The listing builds one solid part. Answer for the finished solid, in the listing's coordinates (mm). Coordinates: 2 decimals unless noted, no trailing zeros. Loops run counter-clockwise (first coordinate to the right, second up) from the corner with the lowest first, then second, coordinate; pieces in that order, holes last. Notation, with made-up numbers: (33, 3.5) - (61, 3.5) arc R12 cw to (61, 24.5) - close; hole circle Ø1 at (-39, 12.25). An arc over 180 degrees is marked (long way). One line per question, with ' | ' between items.
from build123d import *

# Parameters (mm, degrees)
F0_W     = 6.985
F0_H     = 1.5875
F1_DEPTH = 0.94615
F2_W     = 1.5875
F2_H     = 1.5875
F3_DEPTH = 4.445
F4_R     = 0.762


with BuildPart() as f1:
    # F0 (on Top) → F1 (new body)
    with BuildSketch(Plane.XY):
        with Locations((3.4925, 0.79375)):
            Rectangle(F0_W, F0_H)
    extrude(amount=F1_DEPTH)

    # F2 (on face) → F3 (join)
    with BuildSketch(Plane.XY.offset(0.94615)):
        with Locations((0.79375, 0.79375)):
            Rectangle(F2_W, F2_H)
        with Locations((6.19125, 0.79375)):
            Rectangle(F2_W, F2_H)
    extrude(amount=F3_DEPTH)

    # F4
    f4_edges = [f1.edges().sort_by_distance(p)[0] for p in [
        (0, 0, 2.695575),
        (1.5875, 0, 3.16865),
        (3.4925, 0, 0.94615),
        (5.3975, 0, 3.16865),
        (6.985, 0, 2.695575),
        (0, 1.5875, 2.695575),
        (1.5875, 1.5875, 3.16865),
        (3.4925, 1.5875, 0.94615),
        (5.3975, 1.5875, 3.16865),
        (6.985, 1.5875, 2.695575),
    ]]
    fillet(f4_edges, radius=F4_R)


solid = f1.part
Item 1: Find section C-C, the plane x = 4.5. Write down the section's boundary in (y, z), plus the area to 3 significant figures.
Taken from the geometry:
outline: (0, 0) - (1.59, 0) - (1.59, 0.18) arc R0.76 ccw to (0.83, 0.95) - (0.76, 0.95) arc R0.76 ccw to (0, 0.18) - close | area: 1.25 mm2
Item 2: Find section B-B, the plane y = 0.55. Write down the section's boundary in (x, z).
Taken from the geometry:
outline: (0.03, 0) - (6.95, 0) - (6.95, 5.39) - (5.43, 5.39) - (5.43, 0.92) - (1.56, 0.92) - (1.56, 5.39) - (0.03, 5.39) - close
Item 3: Find the intervals of material crossed by line 1 (X direction, y = 0.75, z = 4.8); line 2 (X direction, y = 1.4, z = 3.2); line 3 (Z direction, x = 3.5, y = 0.7), in increasing order. Write a range as [from, to].
Taken from the geometry:
line 1: x = [0, 1.59], [5.4, 6.98] | line 2: x = [0.26, 1.33], [5.66, 6.72] | line 3: z = [0, 0.94]
